Verification items for the finished model (mm, model axes). A direction names the side the tool comes from. Round coordinates to 2 decimals unless told otherwise and drop trailing zeros. Order: outer loops, then holes, each group sorted by start corner. A loop starts at its lowest first (then second) coordinate and runs counter-clockwise, first axis right, second up. Notation, with made-up numbers: M 36.25,41 L 70.25,41 A8 cw 70.25,49 Z; hole C 71,81.5 d8. An arc over 180 degrees is marked long. Answer as a JSON object with one key per item and string values. Group by question number.
```python
from build123d import *

# Parameters (mm, degrees)
SKETCH1_W               = 25.4
SKETCH1_H               = 25.4
SKETCH1_W_2             = 22.225
SKETCH1_H_2             = 22.225
BOSS_EXTRUDE1_DEPTH     = 838.2
SKETCH3_R               = 2.54
SKETCH3_R_2             = 3.429
CUT_EXTRUDE2_DEPTH      = 839.969343898
CUT_EXTRUDE3_DEPTH      = 839.969343898
CUT_EXTRUDE3_DEPTH_BACK = 839.969343898
SKETCH4_R               = 6.604


with BuildPart() as part:
    # Sketch1 → Boss-Extrude1 (new body)
    with BuildSketch(Plane.XY):
        with Locations((12.7, 12.7)):
            Rectangle(SKETCH1_W, SKETCH1_H)
        with Locations((12.7, 12.7)):
            Rectangle(SKETCH1_W_2, SKETCH1_H_2, mode=Mode.SUBTRACT)
    extrude(amount=BOSS_EXTRUDE1_DEPTH)

    # Sketch3 → Cut-Extrude2 (cut, through all)
    with BuildSketch(Plane(origin=(0, 25.4, 0), x_dir=(1, 0, 0), z_dir=(0, 1, 0))):
        with Locations(Location((12.7, -12.7, 0), (0, 0, 270))):
            Circle(SKETCH3_R)
        with Locations(Location((12.7, -825.5, 0), (0, 0, 270))):
            Circle(SKETCH3_R)
        with Locations(Location((12.7, -38.1, 0), (0, 0, 270))):
            Circle(SKETCH3_R)
        with Locations(Location((12.7, -88.9, 0), (0, 0, 270))):
            Circle(SKETCH3_R_2)
        with Locations(Location((12.7, -800.1, 0), (0, 0, 270))):
            Circle(SKETCH3_R)
        with Locations(Location((12.7, -774.7, 0), (0, 0, 270))):
            Circle(SKETCH3_R)
        with Locations(Location((12.7, -749.3, 0), (0, 0, 270))):
            Circle(SKETCH3_R)
    extrude(amount=-CUT_EXTRUDE2_DEPTH, mode=Mode.SUBTRACT)

    # Sketch4 → Cut-Extrude3 (cut, two sides: drawn at the far end of the back side and taken through both)
    with BuildSketch(Plane(origin=(25.4, 0, 0), x_dir=(0, 0, -1), z_dir=(1, 0, 0)).offset(-CUT_EXTRUDE3_DEPTH_BACK)):
        with Locations(Location((-812.8, 12.7, 0), (0, 0, 180))):
            Circle(SKETCH4_R)
    extrude(amount=CUT_EXTRUDE3_DEPTH + CUT_EXTRUDE3_DEPTH_BACK, mode=Mode.SUBTRACT)


solid = part.part
```
Q1. Thickness scan on line 1 (Y direction, x = 8.25, z = 604.5); line 2 (X direction, y = 0.7, z = 800.1). Record the ranges inside material, lowest first. Write a range as from..to.
Q2. Tool access check on faces 5 (the face through (1, 13, 0)), 6 (the face through (13, 23.812, 413)). Record the directions out of +Z, -Z, +X, -X, +Y, -Y that give a thin tool (end or side, any length) a straight path to the whole face; none if there is none.
Q3. Gauge pin test, flat end, axial feed: pin 1 Ø4 at (x, y) = (19.5, 4.5) entering from -Z. Record the tip position at first contact, or that the pin passes through.
Q4. Release check for a two-part mould opening along Y. For faces 1 (the face through (0.78, 16.72, 807.56)), 2 (the face through (13, 25.4, 413)), 3 (the face through (13, 0, 413)), 4 (the face through (25.4, 13, 413)) record: released by +Y, released by -Y, zero draft, split by the parting line, or undercut.
Q5. Cross-section at A-A, the plane z = 67. Record the cut outline in (x, y).
Conclusion:
{
 "1": {"line 1": "0..1.59, 23.81..25.4", "line 2": "0..10.16, 15.24..25.4"},
 "2": {"face 5": "-Z, +X, -X, +Y, -Y", "face 6": "+Z, -Z"},
 "3": {"pin 1": "through"},
 "4": {"face 1": "undercut", "face 2": "released by +Y", "face 3": "released by -Y", "face 4": "zero draft"},
 "5": {"outline": "M 0,0 L 25.4,0 L 25.4,25.4 L 0,25.4 Z; hole M 1.59,1.59 L 23.81,1.59 L 23.81,23.81 L 1.59,23.81 Z"}
}
